from build123d import *

# Parameters (mm, degrees)
SKETCH1_W               = 65
SKETCH1_H               = 60
BOSS_EXTRUDE1_DEPTH     = 10
SKETCH6_W               = 10
SKETCH6_H               = 1
BOSS_EXTRUDE6_DEPTH     = 1
CUT_EXTRUDE2_DEPTH      = 1
CUT_EXTRUDE2_DEPTH_BACK = 73.945184899
BOSS_EXTRUDE2_DEPTH     = 33
SKETCH2_W               = 20.25
SKETCH2_H               = 52.5
CUT_EXTRUDE1_DEPTH      = 100.569071503
BOSS_EXTRUDE3_DEPTH     = 7.5
SKETCH5_W               = 85
SKETCH5_H               = 7.611423687
BOSS_EXTRUDE5_DEPTH     = 70
SKETCH8_W               = 65
SKETCH8_H               = 22.888576313
CUT_EXTRUDE3_DEPTH      = 2
CUT_EXTRUDE4_DEPTH      = 2
SKETCH11_W              = 7
SKETCH11_H              = 60
CUT_EXTRUDE5_DEPTH      = 12.75
CUT_EXTRUDE6_REACH      = 93.359
SKETCH10_W              = 15
SKETCH10_H              = 8
FILLET1_R               = 2
BOSS_EXTRUDE7_START     = 4.5
BOSS_EXTRUDE7_DEPTH     = 4.5
CUT_EXTRUDE8_REACH      = 96.851


with BuildPart() as part:
    # Sketch1 → Boss-Extrude1 (new body)
    with BuildSketch(Plane.XY):
        Rectangle(SKETCH1_W, SKETCH1_H)
        Polygon((32.5, -30), (32.5, 30), (-32.5, 30), (-32.5, -30), (-42.5, -30), (-42.5, 40), (42.5, 40), (42.5, -30), align=None)
    extrude(amount=BOSS_EXTRUDE1_DEPTH)

    # Sketch6 → Boss-Extrude6 (add)
    with BuildSketch(Plane.XY.offset(10)):
        with Locations((12.5, 17)):
            Rectangle(SKETCH6_W, SKETCH6_H)
        with Locations((-12.5, 17)):
            Rectangle(SKETCH6_W, SKETCH6_H)
    extrude(amount=BOSS_EXTRUDE6_DEPTH)

    # Sketch7 → Cut-Extrude2 (cut, two sides: drawn at the far end of the back side and taken through both)
    with BuildSketch(Plane(origin=(17.5, 0, 0), x_dir=(0, 0, -1), z_dir=(1, 0, 0)).offset(-CUT_EXTRUDE2_DEPTH_BACK)):
        Polygon((-10, 16.5), (-11, 17.5), (-11, 16.5), align=None)
    extrude(amount=CUT_EXTRUDE2_DEPTH + CUT_EXTRUDE2_DEPTH_BACK, mode=Mode.SUBTRACT)

    # Sketch1<3> → Boss-Extrude2 (add)
    with BuildSketch(Plane.XY):
        Polygon((32.5, -30), (32.5, 30), (-32.5, 30), (-32.5, -30), (-42.5, -30), (-42.5, 40), (42.5, 40), (42.5, -30), align=None)
    extrude(amount=BOSS_EXTRUDE2_DEPTH)

    # Sketch2 → Cut-Extrude1 (cut, through all)
    with BuildSketch(Plane.ZY.offset(42.5)):
        with Locations((22.875, -3.75)):
            Rectangle(SKETCH2_W, SKETCH2_H)
    extrude(amount=-CUT_EXTRUDE1_DEPTH, mode=Mode.SUBTRACT)

    # Sketch3 → Boss-Extrude3 (add)
    with BuildSketch(Plane.XY.offset(33)):
        Polygon((32.5, 22.5), (42.5, 22.5), (42.5, 40), (-42.5, 40), (-42.5, 22.5), (-32.5, 22.5), (-32.5, 30), (32.5, 30), align=None)
    extrude(amount=BOSS_EXTRUDE3_DEPTH)

    # Sketch5 → Boss-Extrude5 (add)
    with BuildSketch(Plane(origin=(0, 40, 0), x_dir=(1, 0, 0), z_dir=(0, 1, 0))):
        with Locations((0, -36.694288157)):
            Rectangle(SKETCH5_W, SKETCH5_H)
    extrude(amount=-BOSS_EXTRUDE5_DEPTH)

    # Sketch8 → Cut-Extrude3 (cut)
    with BuildSketch(Plane.XZ.offset(-30)):
        with Locations((0, 21.444288157)):
            Rectangle(SKETCH8_W, SKETCH8_H)
    extrude(amount=-CUT_EXTRUDE3_DEPTH, mode=Mode.SUBTRACT)

    # Sketch9 → Cut-Extrude4 (cut)
    with BuildSketch(Plane.ZY.offset(-32.5)):
        Polygon((32.888576313, 22.5), (32.888576313, 32), (10, 32), (10, -30), (12.75, -30), (12.75, 22.5), align=None)
    cut_extrude4 = extrude(amount=-CUT_EXTRUDE4_DEPTH, mode=Mode.SUBTRACT)

    # Mirror1: Cut-Extrude4 across plane
    add(cut_extrude4.mirror(Plane(origin=(0, 0, 0), x_dir=(0, 0, 1), z_dir=(1, 0, 0))), mode=Mode.SUBTRACT)

    # Sketch11 → Cut-Extrude5 (cut)
    with BuildSketch(Plane(origin=(0, 0, 0), x_dir=(-1, 0, 0), z_dir=(0, 0, -1))):
        with Locations((-19, 0)):
            Rectangle(SKETCH11_W, SKETCH11_H)
    cut_extrude5 = extrude(amount=-CUT_EXTRUDE5_DEPTH, mode=Mode.SUBTRACT)

    # Mirror2: Cut-Extrude5 across plane
    add(cut_extrude5.mirror(Plane(origin=(0, 0, 0), x_dir=(0, 0, 1), z_dir=(1, 0, 0))), mode=Mode.SUBTRACT)

    # Sketch10 → Cut-Extrude6 (cut, up to next)
    with BuildSketch(Plane(origin=(0, 40, 0), x_dir=(1, 0, 0), z_dir=(0, 1, 0)), mode=Mode.PRIVATE) as cut_extrude6_sk1:
        with Locations((12, -25)):
            Rectangle(SKETCH10_W, SKETCH10_H)
    cut_extrude6_tool1 = extrude(cut_extrude6_sk1.sketch, amount=-CUT_EXTRUDE6_REACH, mode=Mode.PRIVATE) & part.part
    cut_extrude6 = cut_extrude6_tool1.solids().sort_by_distance((12, 40, 25))[0]
    add(cut_extrude6, mode=Mode.SUBTRACT)

    # Mirror4: Cut-Extrude6 across plane
    add(cut_extrude6.mirror(Plane(origin=(0, 0, 0), x_dir=(0, 0, 1), z_dir=(1, 0, 0))), mode=Mode.SUBTRACT)

    # Fillet1
    fillet1_edges = [part.edges().sort_by_distance(p)[0] for p in [
        (42.5, -3.75, 12.75),
        (-42.5, -3.75, 12.75),
        (42.5, 5, 40.5),
        (-42.5, 5, 40.5),
        (-42.5, -3.75, 32.888576313),
        (42.5, -3.75, 32.888576313),
        (34.5, -3.75, 12.75),
        (-34.5, -3.75, 12.75),
        (4.5, 36, 29),
        (4.5, 36, 21),
        (19.5, 36, 21),
        (19.5, 36, 29),
        (-4.5, 36, 21),
        (-4.5, 36, 29),
        (-19.5, 36, 29),
        (-19.5, 36, 21),
        (-42.5, 5, 0),
        (42.5, 5, 0),
    ]]
    fillet(fillet1_edges, radius=FILLET1_R)

    # Sketch12 → Boss-Extrude7 (add)
    with BuildSketch(Plane.XZ.offset(30).offset(BOSS_EXTRUDE7_START)):
        with BuildLine():
            Line((-42.5, 38.5), (-42.5, 34.888576313))
            ThreePointArc((-42.5, 34.888576313), (-41.914213562, 33.474362751), (-40.5, 32.888576313))
            Line((-40.5, 32.888576313), (40.5, 32.888576313))
            ThreePointArc((40.5, 32.888576313), (41.914213562, 33.474362751), (42.5, 34.888576313))
            Line((42.5, 34.888576313), (42.5, 38.5))
            ThreePointArc((42.5, 38.5), (41.914213562, 39.914213562), (40.5, 40.5))
            Line((40.5, 40.5), (-40.5, 40.5))
            ThreePointArc((-40.5, 40.5), (-41.914213562, 39.914213562), (-42.5, 38.5))
        make_face()
    extrude(amount=-BOSS_EXTRUDE7_DEPTH)

    # Sketch14 → Cut-Extrude8 (cut, up to next)
    with BuildSketch(Plane(origin=(0, 40, 0), x_dir=(1, 0, 0), z_dir=(0, 1, 0)), mode=Mode.PRIVATE) as cut_extrude8_sk1:
        with BuildLine():
            Line((17.5, -18), (6.5, -18))
            ThreePointArc((6.5, -18), (2.964466094, -19.464466094), (1.5, -23))
            Line((1.5, -23), (1.5, -27))
            ThreePointArc((1.5, -27), (2.964466094, -30.535533906), (6.5, -32))
            Line((6.5, -32), (17.5, -32))
            ThreePointArc((17.5, -32), (21.035533906, -30.535533906), (22.5, -27))
            Line((22.5, -27), (22.5, -23))
            ThreePointArc((22.5, -23), (21.035533906, -19.464466094), (17.5, -18))
        make_face()
        with BuildLine():
            Line((19.5, -27), (19.5, -23))
            ThreePointArc((19.5, -23), (18.914213562, -21.585786438), (17.5, -21))
            Line((17.5, -21), (6.5, -21))
            ThreePointArc((6.5, -21), (5.085786438, -21.585786438), (4.5, -23))
            Line((4.5, -23), (4.5, -27))
            ThreePointArc((4.5, -27), (5.085786438, -28.414213562), (6.5, -29))
            Line((6.5, -29), (17.5, -29))
            ThreePointArc((17.5, -29), (18.914213562, -28.414213562), (19.5, -27))
        make_face(mode=Mode.SUBTRACT)
    cut_extrude8_tool1 = extrude(cut_extrude8_sk1.sketch, amount=-CUT_EXTRUDE8_REACH, mode=Mode.PRIVATE) & part.part
    # Sketch14 → Cut-Extrude8 (cut, up to next)
    with BuildSketch(Plane(origin=(0, 40, 0), x_dir=(1, 0, 0), z_dir=(0, 1, 0)), mode=Mode.PRIVATE) as cut_extrude8_sk2:
        with BuildLine():
            Line((-1.5, -23), (-1.5, -27))
            ThreePointArc((-1.5, -27), (-2.964466094, -30.535533906), (-6.5, -32))
            Line((-6.5, -32), (-17.5, -32))
            ThreePointArc((-17.5, -32), (-21.035533906, -30.535533906), (-22.5, -27))
            Line((-22.5, -27), (-22.5, -23))
            ThreePointArc((-22.5, -23), (-21.035533906, -19.464466094), (-17.5, -18))
            Line((-17.5, -18), (-6.5, -18))
            ThreePointArc((-6.5, -18), (-2.964466094, -19.464466094), (-1.5, -23))
        make_face()
        with BuildLine():
            Line((-6.5, -29), (-17.5, -29))
            ThreePointArc((-17.5, -29), (-18.914213562, -28.414213562), (-19.5, -27))
            Line((-19.5, -27), (-19.5, -23))
            ThreePointArc((-19.5, -23), (-18.914213562, -21.585786438), (-17.5, -21))
            Line((-17.5, -21), (-6.5, -21))
            ThreePointArc((-6.5, -21), (-5.085786438, -21.585786438), (-4.5, -23))
            Line((-4.5, -23), (-4.5, -27))
            ThreePointArc((-4.5, -27), (-5.085786438, -28.414213562), (-6.5, -29))
        make_face(mode=Mode.SUBTRACT)
    cut_extrude8_tool2 = extrude(cut_extrude8_sk2.sketch, amount=-CUT_EXTRUDE8_REACH, mode=Mode.PRIVATE) & part.part
    add(cut_extrude8_tool1.solids().sort_by_distance((12, 40, 18.252389))[0], mode=Mode.SUBTRACT)
    add(cut_extrude8_tool2.solids().sort_by_distance((-1.752389, 40, 25))[0], mode=Mode.SUBTRACT)


solid = part.part
Can you work these out from the model? Positions are in its coordinate system, mm. A direction names the side the tool comes from. Round coordinates to 2 decimals unless told otherwise and drop trailing zeros. Loops run counter-clockwise (first coordinate to the right, second up) from the corner with the lowest first, then second, coordinate; pieces in that order, holes last. Notation, with made-up numbers: (42, 67) - (47, 67) arc R23 ccw to (47, 104) - close; hole circle Ø5 at (13.25, -29.5). An arc over 180 degrees is marked (long way). Answer in a Markdown table with one row per item. Add a question column.
Q1. Which directions (+Z, -Z, +X, -X, +Y, -Y) give clear straight access to the entire face, cutting with the end or side of a thin tool? Please do faces 4 (the flat face through (0, -30, 5)), 5 (the flat face through (19, 30, 5)), 6 (the cylindrical face through (-21.07, 36.06, 19.5)), 7 (the cylindrical face through (-41.93, -6.4, 33.49)).
Q2. I want a section at C-C on z = 26. List the corners of the cut face in (x, y) for me.
Q3. I want a section at D-D on z = 5.5. List the corners of the cut face in (x, y) for me, and give its area (3 significant figures).
Q4. I want a section at B-B on x = 13.5. List the corners of the cut face in (y, z) for me.
Q5. For pin 1 Ø2.5 at (x, z) = (-39.5, 24) entering from -Y; pin 2 Ø2 at (x, z) = (-18.5, 4.5) entering from -Y; pin 3 Ø7 at (y, z) = (-14.5, 18) entering from -X, each with a flat end and sliding along its axis, tell me the tip position at first contact or that it passes through.
Q6. I want a section at A-A on y = -5. Count the separate pieces of the cut face and the enclosed holes in it, and give its area (3 significant figures).
Q7. I need wall thicknesses on L1, parallel to X at y = -13, z = 8.5; L2, parallel to X at y = 29, z = 28.5; L3, parallel to Z at x = 1, y = -10.5. Which ranges of each line are inside material? Lowest first, please.
Q8. We'd pull the mould along Z, two halves only. Please class faces 1 (the cylindrical face through (41.93, 4.51, 0.6)), 2 (the flat face through (-19, 30, 5)), 3 (the flat face through (12, 36, 18)): pulls with the +Z half, pulls with the -Z half, needs draft (parallel to the pull), parting line crosses it, or undercut.
A:
| question | item | result |
|---|---|---|
| 1 | face 4 | -Z, +X, -X, -Y |
| 1 | face 5 | -Z, -Y |
| 1 | face 6 | +Y, -Y |
| 1 | face 7 | -X, -Y |
| 2 | outline | (-42.5, 22.5) - (-34.5, 22.5) - (-34.5, 32) - (-22.5, 32) - (-22.5, 40) - (-42.5, 40) - close; (-1.5, 32) - (1.5, 32) - (1.5, 40) - (-1.5, 40) - close; (22.5, 32) - (34.5, 32) - (34.5, 22.5) - (42.5, 22.5) - (42.5, 40) - (22.5, 40) - close |
| 3 | outline | (-42.5, -30) - (-22.5, -30) - (-22.5, 30) - (-15.5, 30) - (-15.5, -30) - (15.5, -30) - (15.5, 30) - (22.5, 30) - (22.5, -30) - (42.5, -30) - (42.5, 40) - (-42.5, 40) - close |
| 3 | area | 5,110 mm^2 |
| 4 | outline | (-34.5, 32.89) - (32, 32.89) - (32, 32) - (40, 32) - (40, 40.5) - (-34.5, 40.5) - close; (-30, 0) - (40, 0) - (40, 18) - (32, 18) - (32, 10) - (17.5, 10) - (17.5, 11) - (16.5, 10) - (-30, 10) - close |
| 5 | pin 1 | y = 22.5 |
| 5 | pin 2 | y = 30 |
| 5 | pin 3 | through |
| 6 | separate pieces | 4 |
| 6 | enclosed holes | 0 |
| 6 | area | 1,390 mm^2 |
| 7 | L1 | -42.5 to -22.5, -15.5 to 15.5, 22.5 to 42.5 |
| 7 | L2 | -42.5 to -34.5, 34.5 to 42.5 |
| 7 | L3 | 0 to 10, 32.89 to 40.5 |
| 8 | face 1 | pulls with the -Z half |
| 8 | face 2 | needs draft |
| 8 | face 3 | undercut |
